Input: part model. Units: mm. Frame: model coordinates. A direction names the side the tool comes from. Give positions to 0.01 mm unless a question says otherwise; leave off trailing zeros. Loops run counter-clockwise (first coordinate to the right, second up) from the corner with the lowest first, then second, coordinate; pieces in that order, holes last. Notation, with made-up numbers: M 79,-8 L 101,-8 A14 cw 101,6 Z; hole C 63,35 d4. An arc over 180 degrees is marked long. Answer as a JSON object with one key per item and string values. Group by question number.
1) Section query C-C on x = 66.5. Return loops of the section in (y, z).
2) First-contact query: P1, Ø0.8, axis at y = 1.5, z = -80.5, coming from the +X side; P2, Ø1, axis at y = 2.5, z = -141.5, coming from the +X side; P3, Ø2, axis at x = 69, z = -81.5, coming from the -Y side; P4, Ø0.9, axis at x = 75, y = 1, coming from the -Z side. Flat tips, straight axial feed; report the tip coordinate or a pass-through.
3) Access query for faces 5 (the flat face through (84.062, 1.479, -93.307)), 6 (the flat face through (73, 1, -95.641)), 7 (the flat face through (-4.561, 1.479, -93.666)), 8 (the cylindrical face through (79.357, 1.479, -91.423)). Directions: +Z, -Z, +X, -X, +Y, -Y. A direction counts if a zero-diameter tool reaches every point of the face in a straight line with its end or side. Return the directions, or none.
4) Ray query, L1, parallel to X at y = 1.7, z = -97; L2, parallel to X at y = 1.05, z = -92.5; L3, parallel to X at y = 0.7, z = -73.5. Return the intervals inside material, ascending.
5) Draft query along Z for faces 1 (the flat face through (24.493, 1.479, -58.659)), 2 (the cylindrical face through (90.844, 1.521, -77.135)), 3 (the flat face through (83.685, 1.479, -90.263)), 4 (the flat face through (29.9, 1.5, -80.1)). Return one class per face: +Z half, -Z half, draft (parallel to the pull), parting line (faces both ways), or undercut.
6) Section query A-A on z = -76. Return loops of the section in (x, y).
7) Section query B-B on x = 26. Return loops of the section in (y, z).
from build123d import *

# Parameters (mm, degrees)
BOSS_EXTRUDE2_DEPTH = 3
FILLET1_R           = 1
FILLET2_R           = 4
FILLET3_R           = 40
FILLET4_R           = 2
FILLET5_R           = 1.4
FILLET6_R           = 30
FILLET7_R           = 3
FILLET8_R           = 6


with BuildPart() as part:
    # Sketch4 → Boss-Extrude2 (new body)
    with BuildSketch(Plane(origin=(0, 0, 0), x_dir=(1, 0, 0), z_dir=(0, 1, 0))):
        with BuildLine():
            Line((87.31, 79.61), (91.618486592, 77.887634392))
            ThreePointArc((91.618486592, 77.887634392), (88.863922918, 68.889748023), (81.855760182, 62.61))
            ThreePointArc((81.855760182, 62.61), (59.656820918, 67.258748235), (39.555721251, 56.754008505))
            Line((39.555721251, 56.754008505), (32.499176634, 60.570465889))
            Line((32.499176634, 60.570465889), (16.517315238, 56.754008505))
            Line((16.517315238, 56.754008505), (7.414760931, 60.570465889))
            Line((7.414760931, 60.570465889), (1.892511031, 56.754008505))
            Line((1.892511031, 56.754008505), (0.46321022, 62.992365596))
            Line((0.46321022, 62.992365596), (9.066007765, 67.967785451))
            Line((9.066007765, 67.967785451), (3.879350061, 108.84040305))
            ThreePointArc((3.879350061, 108.84040305), (2.01611376, 105.85998951), (0.66321022, 102.615892348))
            Line((0.66321022, 102.615892348), (3.879350061, 93.591357519))
            Line((3.879350061, 93.591357519), (-2.93678978, 90.505813501))
            Line((-2.93678978, 90.505813501), (-5.768910997, 92.808331559))
            Line((-5.768910997, 92.808331559), (-1.778138145, 95.640627614))
            Line((-1.778138145, 95.640627614), (-4.765318246, 100.408264948))
            Line((-4.765318246, 100.408264948), (-9.496065378, 101.269350579))
            Line((-9.496065378, 101.269350579), (-6.815233616, 106.290541956))
            Line((-6.815233616, 106.290541956), (-13.555482626, 112.676963609))
            Line((-13.555482626, 112.676963609), (-11.418327461, 116.805813501))
            Line((-11.418327461, 116.805813501), (-6.221647651, 113.305813501))
            ThreePointArc((-6.221647651, 113.305813501), (-4.139581192, 113.712014511), (-4.545782202, 115.79408097))
            Line((-4.545782202, 115.79408097), (-10.724979751, 119.955813501))
            Line((-10.724979751, 119.955813501), (-8.365992616, 124.387469749))
            Line((-8.365992616, 124.387469749), (-2.93678978, 123.666991194))
            Line((-2.93678978, 123.666991194), (-2.93678978, 130.055848545))
            Line((-2.93678978, 130.055848545), (3.413077147, 137.08559026))
            Line((3.413077147, 137.08559026), (0.522809133, 139.95641446))
            Line((0.522809133, 139.95641446), (3.698074275, 147.318161123))
            ThreePointArc((3.698074275, 147.318161123), (3.364070449, 150.092913281), (0.66321022, 150.811357519))
            Line((0.66321022, 150.811357519), (-1.778138145, 148.370009154))
            Line((-1.778138145, 148.370009154), (-4.999762187, 152.301948586))
            ThreePointArc((-4.999762187, 152.301948586), (-1.941119995, 156.054428227), (2.78321022, 157.111357519))
            ThreePointArc((2.78321022, 157.111357519), (8.815996079, 151.282158066), (11.096791577, 143.209237691))
            ThreePointArc((11.096791577, 143.209237691), (12.311774437, 133.113784868), (6.46321022, 124.795813501))
            Line((6.46321022, 124.795813501), (24.42321022, 92.530161433))
            Line((24.42321022, 92.530161433), (24.42321022, 79.395813501))
            Line((24.42321022, 79.395813501), (35.622369927, 80.833234121))
            Line((35.622369927, 80.833234121), (62.451437904, 95.640627614))
            Line((62.451437904, 95.640627614), (76.661791259, 95.640627614))
            Line((76.661791259, 95.640627614), (80.884676882, 99.013707758))
            Line((80.884676882, 99.013707758), (87.938365698, 101.231357519))
            Line((87.938365698, 101.231357519), (87.31, 93.591357519))
            Line((87.31, 93.591357519), (80.722672152, 93.01504101))
            ThreePointArc((80.722672152, 93.01504101), (79.359113719, 91.390015348), (80.984139381, 90.026456915))
            Line((80.984139381, 90.026456915), (86.46321022, 90.505813501))
            Line((86.46321022, 90.505813501), (85.632866314, 84))
            Line((85.632866314, 84), (81.389705108, 71.508585308))
            ThreePointArc((81.389705108, 71.508585308), (82.327545423, 69.605835839), (84.230294892, 70.543676154))
            Line((84.230294892, 70.543676154), (87.31, 79.61))
        make_face()
    extrude(amount=BOSS_EXTRUDE2_DEPTH)

    # Fillet1
    fillet1_edges = [part.edges().sort_by_distance(p)[0] for p in [
        (3.879350061, 1.5, -108.84040305),
        (-9.496065378, 1.5, -101.269350579),
        (-2.93678978, 1.5, -123.666991194),
    ]]
    fillet(fillet1_edges, radius=FILLET1_R)

    # Fillet2
    fillet2_edges = [part.edges().sort_by_distance(p)[0] for p in [
        (39.555721251, 1.5, -56.754008505),
        (32.499176634, 1.5, -60.570465889),
        (16.517315238, 1.5, -56.754008505),
        (7.414760931, 1.5, -60.570465889),
        (0.46321022, 1.5, -62.992365596),
        (0.66321022, 1.5, -102.615892348),
        (3.879350061, 1.5, -93.591357519),
        (-2.93678978, 1.5, -90.505813501),
        (-4.765318246, 1.5, -100.408264948),
        (-2.93678978, 1.5, -130.055848545),
        (2.78321022, 1.5, -157.111357519),
        (80.884676882, 1.5, -99.013707758),
        (91.618486592, 1.5, -77.887634392),
        (81.855760182, 1.5, -62.61),
    ]]
    fillet(fillet2_edges, radius=FILLET2_R)

    # Fillet3
    fillet3_edges = [part.edges().sort_by_distance(p)[0] for p in [
        (24.42321022, 1.5, -92.530161433),
    ]]
    fillet(fillet3_edges, radius=FILLET3_R)

    # Fillet4
    fillet4_edges = [part.edges().sort_by_distance(p)[0] for p in [
        (9.066007765, 1.5, -67.967785451),
        (-1.778138145, 1.5, -95.640627614),
        (-6.815233616, 1.5, -106.290541956),
        (-8.365992616, 1.5, -124.387469749),
        (6.46321022, 1.5, -124.795813501),
    ]]
    fillet(fillet4_edges, radius=FILLET4_R)

    # Fillet5
    fillet5_edges = [part.edges().sort_by_distance(p)[0] for p in [
        (3.413077147, 1.5, -137.08559026),
        (0.522809133, 1.5, -139.95641446),
        (-4.999762187, 1.5, -152.301948586),
    ]]
    fillet(fillet5_edges, radius=FILLET5_R)

    # Fillet6
    fillet6_edges = [part.edges().sort_by_distance(p)[0] for p in [
        (62.451437904, 1.5, -95.640627614),
    ]]
    fillet(fillet6_edges, radius=FILLET6_R)

    # Fillet7
    fillet7_edges = [part.edges().sort_by_distance(p)[0] for p in [
        (87.938365698, 1.5, -101.231357519),
    ]]
    fillet(fillet7_edges, radius=FILLET7_R)

    # Fillet8
    fillet8_edges = [part.edges().sort_by_distance(p)[0] for p in [
        (-13.555482626, 1.5, -112.676963609),
    ]]
    fillet(fillet8_edges, radius=FILLET8_R)


solid = part.part
Output:
{
 "1": {"outline": "M 0,-95.41 L 3,-95.41 L 3,-67.5 L 0,-67.5 Z"},
 "2": {"P1": "stops at x = 84.58", "P2": "stops at x = 12.03", "P3": "stops at y = 0", "P4": "stops at z = -95.64"},
 "3": {"face 5": "+X, +Y, -Y", "face 6": "-Z, +Y, -Y", "face 7": "-X, +Y, -Y", "face 8": "+Y, -Y"},
 "4": {"L1": "x = -2.65 to 2.66, 5.38 to 21.56, 78.36 to 87.58", "L2": "x = -5.39 to 1.25, 5.95 to 23.06, 56.82 to 79.72", "L3": "x = 8.36 to 82.07, 85.23 to 90.94"},
 "5": {"face 1": "+Z half", "face 2": "parting line", "face 3": "undercut", "face 4": "-Z half"},
 "6": {"outline": "M 8.05,0 L 82.92,0 L 82.92,3 L 8.05,3 Z; M 86.08,0 L 91.22,0 L 91.22,3 L 86.08,3 Z"},
 "7": {"outline": "M 0,-79.6 L 3,-79.6 L 3,-59.02 L 0,-59.02 Z"}
}
